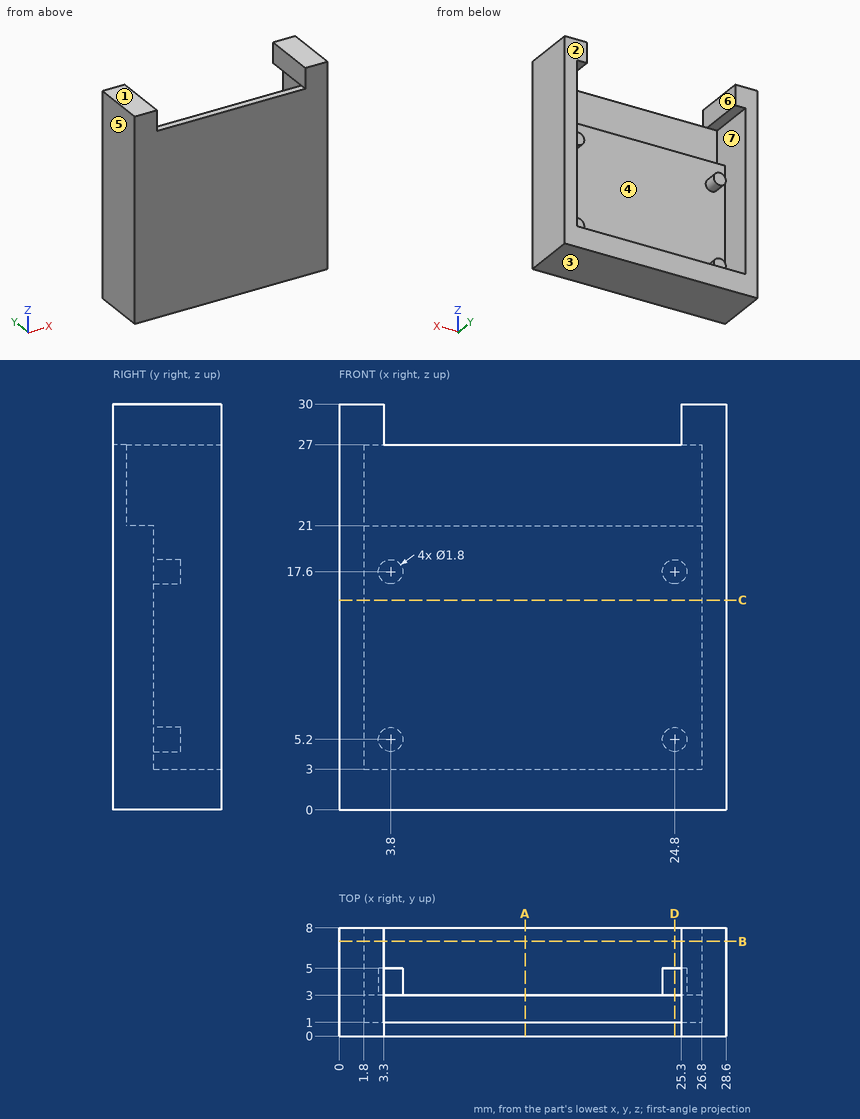
Study the drawing (mm; zero at the part's minimum x, y, z) and answer. A direction names the side the tool comes from. Coordinates: 2 decimals unless noted, no trailing zeros. Write each loop counter-clockwise with the first axis right and the second up, starting at its lowest first coordinate (ties: lowest second). Pieces come first, ordered by that corner, then holes. Notation, with made-up numbers: M -3.75,87 L 25.25,87 A12 ccw 25.25,104 Z; hole C -35.75,64 d10. An arc over 180 degrees is marked long. Use a Markdown table: item, result. Add a question column.
1. Section A-A (x = 13.75) is taken. Give the vertices of the cut face in (y, z).
2. Section D-D (x = 24.8) is taken. Give the vertices of the cut face in (y, z), plus the area to 3 significant figures.
3. Section C-C (z = 15.5) is taken. Give the vertices of the cut face in (x, y).
4. Which of the six approach directions +Z, -Z, +X, -X, +Y, -Y give full straight-line access (tool end or side, diameter ignored) to the marked faces 5, 6 and 7?
5. Given P1, Ø3, axis at x = 8, z = 15.5, coming from the +Y side; P2, Ø2, axis at x = 3.5, z = 18, coming from the +Y side; P3, Ø0.8, axis at x = 17.5, y = 0.5, coming from the +Z side, each flat-ended and moving along its own axis, determine where each tip first touches the part or whether it passes through.
6. Section B-B (y = 7) is taken. Give the vertices of the cut face in (x, z), plus the area to 3 significant figures.
7. Straight lines are drawn through the part: line 1 along X through (y, z) = (3.25, 17.5); line 2 along X through (y, z) = (6.25, 9.75); line 3 along Y through (x, z) = (9.75, 21.25). For each, find the intervals that lie inside material, in ascending order. Write a range as [from, to].
8. For a pull along Z with two mould halves and no side action, classify the marked faces 1, 2, 3 and 4 as +Z half, -Z half, draft (parallel to the pull), parting line (faces both ways), or undercut.
Data:
| question | item | result |
|---|---|---|
| 1 | outline | M 0,0 L 8,0 L 8,3 L 3,3 L 3,21 L 1,21 L 1,27 L 0,27 Z |
| 2 | outline | M 0,0 L 8,0 L 8,3 L 3,3 L 3,4.3 L 5,4.3 L 5,6.1 L 3,6.1 L 3,16.7 L 5,16.7 L 5,18.5 L 3,18.5 L 3,21 L 1,21 L 1,27 L 0,27 Z |
| 2 | area | 91.2 mm2 |
| 3 | outline | M 0,0 L 28.6,0 L 28.6,8 L 26.8,8 L 26.8,3 L 1.8,3 L 1.8,8 L 0,8 Z |
| 4 | face 5 | +Z, -Z, -X, +Y, -Y |
| 4 | face 6 | +Z, +Y, -Y |
| 4 | face 7 | +Y |
| 5 | P1 | stops at y = 3 |
| 5 | P2 | stops at y = 5 |
| 5 | P3 | stops at z = 27 |
| 6 | outline | M 0,0 L 28.6,0 L 28.6,30 L 25.3,30 L 25.3,27 L 26.8,27 L 26.8,3 L 1.8,3 L 1.8,27 L 3.3,27 L 3.3,30 L 0,30 Z |
| 6 | area | 192 mm2 |
| 7 | line 1 | x = [0, 1.8], [2.91, 4.69], [23.91, 25.69], [26.8, 28.6] |
| 7 | line 2 | x = [0, 1.8], [26.8, 28.6] |
| 7 | line 3 | y = [0, 1] |
| 8 | face 1 | +Z half |
| 8 | face 2 | draft |
| 8 | face 3 | -Z half |
| 8 | face 4 | undercut |
